Read the model definition and answer for the solid it produces. Units are mm, in the model's axes. A direction names the side the tool comes from. Coordinates: 2 decimals unless noted, no trailing zeros. Write each loop counter-clockwise with the first axis right and the second up, starting at its lowest first coordinate (ties: lowest second). Pieces come first, ordered by that corner, then holes. Notation, with made-up numbers: (43.5, 49.25) -> (50.5, 49.25) arc R21 ccw to (50.5, 72.25) -> close; hole circle Ø1 at (-12, 52). An arc over 180 degrees is marked (long way). One line per item, written item: value. Start each with the question number.
1. Find section C-C, the plane x = 47.5. Write down the section's boundary in (y, z), and give its area (3 significant figures).
2. Given P1, Ø3.5, axis at x = -5.5, y = -4.75, coming from the -Z side; P2, Ø6.5, axis at x = 47.5, y = -15.25, coming from the -Z side; P3, Ø4, axis at y = -7, z = 26, coming from the -X side; P4, Ø4, axis at y = -10, z = 30.5, coming from the +X side, each flat-ended and moving along its own axis, determine where each tip first touches the part or whether it passes through.
3. Consider line 1 along Y through (x, z) = (47.5, 14.15); line 2 along X through (y, z) = (-14.25, 6); line 3 along Z through (x, y) = (-3.5, -14.5). Determine where each line is inside the solid, lowest interval first.
4. For faces 1 (the cylindrical face through (41.1, -0.86, 27.32)), 2 (the cylindrical face through (12.77, -8.85, -2.71)), 3 (the flat face through (0, -10, 6)), 4 (the cylindrical face through (41.14, -19.1, 27.32)), determine the directions among +Z, -Z, +X, -X, +Y, -Y from which every point of the face is accessible in a straight line to the end or side of a thin tool.
5. Find section B-B, the plane x = 10. Write down the section's boundary in (y, z).
6. Find section A-A, the plane y = -4.75. Write down the section's boundary in (x, z), and give its area (3 significant figures).
7. For a pull along X with two mould halves and no side action, classify faces 5 (the flat face through (10, -10, -5.5)), 6 (the flat face through (42, -10, 27)), 7 (the cylindrical face through (47.76, -13.267, 13.479)), 8 (the cylindrical face through (-5.24, -13.267, 13.479)) as pulls with the +X half, pulls with the -X half, needs draft (parallel to the pull), parting line crosses it, or undercut.
8. Find section D-D, the plane z = 3. Write down the section's boundary in (x, y).
```python
from build123d import *

# Parameters (mm, degrees)
EXTRUDE_1_DEPTH     = 40
EXTRUDE_2_DEPTH     = 3
SKETCH_4_R          = 2
CUT_EXTRUDE_1_DEPTH = 3
SKETCH_5_R          = 3
EXTRUDE_3_DEPTH     = 5.5


with BuildPart() as part:
    # 草图1 → 凸台-拉伸1 (new body)
    with BuildSketch(Plane.XY):
        with BuildLine():
            Line((3, 0), (39, 0))
            ThreePointArc((39, 0), (41.121320344, -0.878679656), (42, -3))
            Line((42, -3), (42, -17))
            ThreePointArc((42, -17), (41.121320344, -19.121320344), (39, -20))
            Line((39, -20), (3, -20))
            ThreePointArc((3, -20), (0.878679656, -19.121320344), (0, -17))
            Line((0, -17), (0, -3))
            ThreePointArc((0, -3), (0.878679656, -0.878679656), (3, 0))
        make_face()
    extrude(amount=EXTRUDE_1_DEPTH)

    # 草图3 → 凸台-拉伸2 (add)
    with BuildSketch(Plane.XY.offset(12)):
        with BuildLine():
            Line((3, 0), (-8, 0))
            Line((-8, 0), (-8, -20))
            Line((-8, -20), (3, -20))
            ThreePointArc((3, -20), (0.878679656, -19.121320344), (0, -17))
            Line((0, -17), (0, -3))
            ThreePointArc((0, -3), (0.878679656, -0.878679656), (3, 0))
        make_face()
        with BuildLine():
            Line((42, -3), (42, -17))
            ThreePointArc((42, -17), (41.121320344, -19.121320344), (39, -20))
            Line((39, -20), (50, -20))
            Line((50, -20), (50, 0))
            Line((50, 0), (39, 0))
            ThreePointArc((39, 0), (41.121320344, -0.878679656), (42, -3))
        make_face()
    extrude(amount=EXTRUDE_2_DEPTH)

    # 草图4 → 切除-拉伸1 (cut)
    with BuildSketch(Plane(origin=(0, 0, 12), x_dir=(-1, 0, 0), z_dir=(0, 0, -1))):
        with Locations((5.5, -4.75)):
            Circle(SKETCH_4_R)
        with Locations((5.5, -15.25)):
            Circle(SKETCH_4_R)
        with Locations((-47.5, -4.75)):
            Circle(SKETCH_4_R)
        with Locations((-47.5, -15.25)):
            Circle(SKETCH_4_R)
    extrude(amount=-CUT_EXTRUDE_1_DEPTH, mode=Mode.SUBTRACT)

    # 草图5 → 凸台-拉伸3 (add)
    with BuildSketch(Plane(origin=(0, 0, 0), x_dir=(-1, 0, 0), z_dir=(0, 0, -1))):
        with Locations(Location((-10, -10, 0), (0, 0, 180))):
            Circle(SKETCH_5_R)
    extrude(amount=EXTRUDE_3_DEPTH)


solid = part.part
```
Answer block:
1. outline: (-20, 12) -> (-17.25, 12) -> (-17.25, 15) -> (-20, 15) -> close; (-13.25, 12) -> (-6.75, 12) -> (-6.75, 15) -> (-13.25, 15) -> close; (-2.75, 12) -> (0, 12) -> (0, 15) -> (-2.75, 15) -> close
1. area: 36.0 mm2
2. P1: passes through
2. P2: stops at z = 12
2. P3: stops at x = 0
2. P4: stops at x = 42
3. line 1: y = -20 to -17.25, -13.25 to -6.75, -2.75 to 0
3. line 2: x = 0 to 42
3. line 3: z = 12 to 15
4. face 1: +Z, +X, +Y
4. face 2: -Z
4. face 3: -Z, -X, +Y, -Y
4. face 4: +Z, +X, -Y
5. outline: (-20, 0) -> (-13, 0) -> (-13, -5.5) -> (-7, -5.5) -> (-7, 0) -> (0, 0) -> (0, 40) -> (-20, 40) -> close
6. outline: (-8, 12) -> (-7.5, 12) -> (-7.5, 15) -> (-8, 15) -> close; (-3.5, 12) -> (0, 12) -> (0, 0) -> (42, 0) -> (42, 12) -> (45.5, 12) -> (45.5, 15) -> (42, 15) -> (42, 40) -> (0, 40) -> (0, 15) -> (-3.5, 15) -> close; (49.5, 12) -> (50, 12) -> (50, 15) -> (49.5, 15) -> close
6. area: 1,700 mm2
7. face 5: needs draft
7. face 6: pulls with the +X half
7. face 7: undercut
7. face 8: undercut
8. outline: (0, -17) arc R3 ccw to (3, -20) -> (39, -20) arc R3 ccw to (42, -17) -> (42, -3) arc R3 ccw to (39, 0) -> (3, 0) arc R3 ccw to (0, -3) -> close
